Geometry check sheet. Reference: the model listing, model coordinates, mm. A direction names the side the tool comes from. Give positions to 0.01 mm unless a question says otherwise; leave off trailing zeros. Write each loop counter-clockwise with the first axis right and the second up, starting at its lowest first coordinate (ties: lowest second). Pieces come first, ordered by that corner, then holes. Notation, with made-up numbers: (72.25, 40.25) - (112.25, 40.25) arc R19 cw to (112.25, 63.25) - close; hole circle Ø10 at (10.5, 2). An arc over 180 degrees is marked (long way). Write item = value, one per line. Start each with the question number.
(1) Depth check by flat-ended pin: pin 1 Ø17 at (x, y) = (7.5, 10) entering from -Z; pin 2 Ø1 at (x, z) = (-2, -4.5) entering from +Y; pin 3 Ø2 at (y, z) = (14.5, 10) entering from +X; pin 4 Ø12 at (x, z) = (9.5, -7) entering from -Y. Enter the tip coordinate at first touch or a pass-through.
(2) Access from +Z, -Z, +X, -X, +Y, -Y to the whole of each face (thin tool, end or side, straight path). Record for faces 1 (the cylindrical face through (-0.491, -2.213, -4.93)), 2 (the flat face through (-20, 0, 20)), 3 (the cylindrical face through (-18.95, -2.01, 14.93)).
(3) Section check A-A, the plane y = 0. Enter the section's corners in (x, z).
(4) Section check C-C, the plane z = 8.25. Enter the section's corners in (x, y), plus the area to 3 significant figures.
(5) Section check D-D, the plane x = -20. Enter the section's corners in (y, z), plus the area to 3 significant figures.
(6) Section check B-B, the plane x = 0. Enter the section's corners in (y, z).
(7) Thickness scan on L1, parallel to Z at x = 18, y = -11.5; L2, parallel to X at y = 16, z = 3; L3, parallel to Y at x = 13, z = 4. Record the ranges inside material, lowest first.
```python
from build123d import *

# Parameters (mm, degrees)
SKETCH1_R           = 28.337466136
SKETCH1_R_2         = 2.266997291
BOSS_EXTRUDE1_DEPTH = 10
SKETCH1_2_R         = 2.266997291
BOSS_EXTRUDE2_DEPTH = 10
SKETCH1_4_R         = 2.266997291
BOSS_EXTRUDE3_DEPTH = 20


with BuildPart() as part:
    # Sketch1 → Boss-Extrude1 (new body)
    with BuildSketch(Plane.XY):
        Circle(SKETCH1_R)
        Circle(SKETCH1_R_2, mode=Mode.SUBTRACT)
        with Locations((-20, 0)):
            Circle(SKETCH1_R_2, mode=Mode.SUBTRACT)
    extrude(amount=BOSS_EXTRUDE1_DEPTH)

    # Sketch1<2> → Boss-Extrude2 (add, symmetric)
    with BuildSketch(Plane.XY):
        Circle(SKETCH1_2_R)
    extrude(amount=BOSS_EXTRUDE2_DEPTH, both=True)

    # Sketch1<4> → Boss-Extrude3 (add)
    with BuildSketch(Plane.XY):
        with Locations((-20, 0)):
            Circle(SKETCH1_4_R)
    extrude(amount=BOSS_EXTRUDE3_DEPTH)


solid = part.part
```
Model answer:
q1.pin_1 = 0
q1.pin_2 = 1.7
q1.pin_3 = 24.92
q1.pin_4 = through
q2.face_1 = -Z
q2.face_2 = +Z, +X, -X, +Y, -Y
q2.face_3 = +Z
q3.outline = (-28.34, 0) - (-2.27, 0) - (-2.27, -10) - (2.27, -10) - (2.27, 0) - (28.34, 0) - (28.34, 10) - (-17.73, 10) - (-17.73, 20) - (-22.27, 20) - (-22.27, 10) - (-28.34, 10) - close
q4.outline = circle Ø56.67 at (0, 0)
q4.area = 2,520 mm²
q5.outline = (-20.08, 0) - (20.08, 0) - (20.08, 10) - (2.27, 10) - (2.27, 20) - (-2.27, 20) - (-2.27, 10) - (-20.08, 10) - close
q5.area = 447 mm²
q6.outline = (-28.34, 0) - (-2.27, 0) - (-2.27, -10) - (2.27, -10) - (2.27, 0) - (28.34, 0) - (28.34, 10) - (-28.34, 10) - close
q7.L1 = 0 to 10
q7.L2 = -23.39 to 23.39
q7.L3 = -25.18 to 25.18
